For this review, take the finished solid that the model builds, in its own axes (mm). Round coordinates to 2 decimals unless told otherwise and drop trailing zeros. Write each loop counter-clockwise with the first axis right and the second up, starting at its lowest first coordinate (ties: lowest second). Pieces come first, ordered by that corner, then holes. Notation, with made-up numbers: M 24,65 L 83,65 A27 ccw 83,89 Z; hole C 25.5,-9.75 d7. An arc over 180 degrees is marked long. Use one line per item in the form item = value. Start each with the question number.
Item 1: For line 1 (Z direction, x = 0, y = 37); line 2 (X direction, y = 8.5, z = 27); line 3 (Y direction, x = -55.5, z = 0), list the stretches that pass through material, from the lowest coordinate up. Write a range as [from, to].
Item 2: Add section C-C (y = 25). State the section outline as (x, z) points, and give its area (3 significant figures).
Item 3: Draft analysis for pull direction X (two halves, no side actions). For faces 1 (the cylindrical face through (56.218, 24.65, -7.381)), 2 (the flat face through (-41.7, 50, 37.5)), 3 (the cylindrical face through (0.195, 26.487, -55.95)), state which applies: released by +X, released by -X, zero draft, split by the parting line, or undercut.
Item 4: Add section A-A (z = 0). State the section outline as (x, y) points.
Item 5: For P1, Ø1.5, axis at x = -1, y = 24.5, coming from the +Z side; P2, Ø2.5, axis at x = 0, y = 25, coming from the -Z side; P3, Ø6, axis at x = -28.5, y = 44.5, coming from the +Z side; P4, Ø1, axis at y = 19, z = -27, coming from the +X side, all flat-tipped, find the tip position at first contact; note any pin that passes through.
Item 6: Add section D-D (y = 33). State the section outline as (x, z) points, and give its area (3 significant figures).
Item 7: Add section B-B (x = 0). State the section outline as (y, z) points.
from build123d import *

# Parameters (mm, degrees)
SKETCH1_R           = 56.7
SKETCH1_R_2         = 55.2
BOSS_EXTRUDE1_DEPTH = 50
FILLET1_R           = 0.5
SKETCH2_R           = 1.5
CUT_EXTRUDE1_DEPTH  = 10
CIRPATTERN1_COUNT   = 4


with BuildPart() as part:
    # Sketch1 → Boss-Extrude1 (new body)
    with BuildSketch(Plane(origin=(0, 0, 0), x_dir=(1, 0, 0), z_dir=(0, 1, 0))):
        with Locations(Location((0, 0, 0), (0, 0, 270))):
            Circle(SKETCH1_R)
        with Locations(Location((0, 0, 0), (0, 0, 270))):
            Circle(SKETCH1_R_2, mode=Mode.SUBTRACT)
    extrude(amount=BOSS_EXTRUDE1_DEPTH)

    # Fillet1
    fillet1_edges = [part.edges().sort_by_distance(p)[0] for p in [
        (0, 0, -55.2),
        (0, 50, -55.2),
    ]]
    fillet(fillet1_edges, radius=FILLET1_R)

    # Sketch2 → Cut-Extrude1 (cut)
    with BuildSketch(Plane(origin=(56.7, 0, 0), x_dir=(0, 0, -1), z_dir=(1, 0, 0))):
        with Locations((0, 25)):
            Circle(SKETCH2_R)
    cut_extrude1 = extrude(amount=-CUT_EXTRUDE1_DEPTH, mode=Mode.SUBTRACT)

    # CirPattern1: Cut-Extrude1 ×4 about axis
    cirpattern1_axis = Axis((0, 48.063508327, 0), (0, -1, 0))
    for i in range(1, CIRPATTERN1_COUNT):
        add(cut_extrude1.rotate(cirpattern1_axis, i * 360 / CIRPATTERN1_COUNT), mode=Mode.SUBTRACT)


solid = part.part
Calculated:
q1.line_1 = [-56.7, -55.2], [55.2, 56.7]
q1.line_2 = [-49.86, -48.15], [48.15, 49.86]
q1.line_3 = [0.04, 23.5], [26.5, 49.96]
q2.outline = M -56.68,-1.5 A56.7 ccw -1.5,-56.68 L -1.5,-55.18 A55.2 cw -55.18,-1.5 Z; M -56.68,1.5 L -55.18,1.5 A55.2 cw -1.5,55.18 L -1.5,56.68 A56.7 ccw Z; M 1.5,-56.68 A56.7 ccw 56.68,-1.5 L 55.18,-1.5 A55.2 cw 1.5,-55.18 Z; M 1.5,55.18 A55.2 cw 55.18,1.5 L 56.68,1.5 A56.7 ccw 1.5,56.68 Z
q2.area = 509 mm^2
q3.face_1 = split by the parting line
q3.face_2 = zero draft
q3.face_3 = undercut
q4.outline = M -56.7,0 L -55.7,0 A0.5 ccw -55.2,0.5 L -55.2,23.5 L -56.7,23.5 Z; M -56.7,26.5 L -55.2,26.5 L -55.2,49.5 A0.5 ccw -55.7,50 L -56.7,50 Z; M 55.2,0.5 A0.5 ccw 55.7,0 L 56.7,0 L 56.7,23.5 L 55.2,23.5 Z; M 55.2,26.5 L 56.7,26.5 L 56.7,50 L 55.7,50 A0.5 ccw 55.2,49.5 Z
q5.P1 = 56.69
q5.P2 = through
q5.P3 = 50.64
q5.P4 = 50.13
q6.outline = C 0,0 d113.4; hole C 0,0 d110.4
q6.area = 527 mm^2
q7.outline = M 0,-56.7 L 23.5,-56.7 L 23.5,-55.2 L 0.5,-55.2 A0.5 ccw 0,-55.7 Z; M 0,55.7 A0.5 ccw 0.5,55.2 L 23.5,55.2 L 23.5,56.7 L 0,56.7 Z; M 26.5,-56.7 L 50,-56.7 L 50,-55.7 A0.5 ccw 49.5,-55.2 L 26.5,-55.2 Z; M 26.5,55.2 L 49.5,55.2 A0.5 ccw 50,55.7 L 50,56.7 L 26.5,56.7 Z
